Geometry check sheet. Reference: the model listing, model coordinates, mm. A direction names the side the tool comes from. Coordinates: 2 decimals unless noted, no trailing zeros. Loops run counter-clockwise (first coordinate to the right, second up) from the corner with the lowest first, then second, coordinate; pieces in that order, holes last.
Autodesk Fusion 360 part; units mm, degrees
sketch "Sketch1" plane through (0, 0, 0) normal (0, 0, 1) x (1, 0, 0)
  line L0 (0, 0) -> (-24.511, 0)
  line L1 (0, 0) -> (-1.1547, 2)
  line L2 (-1.1547, 2) -> (-3.1547, 2)
  line L3 (-3.1547, 2) -> (-4.6106, 6)
  line L4 (-4.6106, 6) -> (-4.9865, 5.8632)
  line L5 (-4.9865, 5.8632) -> (-3.5804, 2)
  line L6 (-3.5804, 2) -> (-4.1547, 2)
  line L7 (-4.5804, 2) -> (-5.1547, 2)
  line L8 (-5.9865, 5.8632) -> (-4.5804, 2)
  line L9 (-5.6106, 6) -> (-5.9865, 5.8632)
  line L10 (-4.1547, 2) -> (-5.6106, 6)
  line L11 (-5.5804, 2) -> (-6.1547, 2)
  line L12 (-6.9865, 5.8632) -> (-5.5804, 2)
  line L13 (-6.6106, 6) -> (-6.9865, 5.8632)
  line L14 (-5.1547, 2) -> (-6.6106, 6)
  line L15 (-6.5804, 2) -> (-7.1547, 2)
  line L16 (-7.9865, 5.8632) -> (-6.5804, 2)
  line L17 (-7.6106, 6) -> (-7.9865, 5.8632)
  line L18 (-6.1547, 2) -> (-7.6106, 6)
  line L19 (-7.5804, 2) -> (-8.1547, 2)
  line L20 (-8.9865, 5.8632) -> (-7.5804, 2)
  line L21 (-8.6106, 6) -> (-8.9865, 5.8632)
  line L22 (-7.1547, 2) -> (-8.6106, 6)
  line L23 (-8.5804, 2) -> (-9.1547, 2)
  line L24 (-9.9865, 5.8632) -> (-8.5804, 2)
  line L25 (-9.6106, 6) -> (-9.9865, 5.8632)
  line L26 (-8.1547, 2) -> (-9.6106, 6)
  line L27 (-9.1547, 2) -> (-12.9865, 2)
  line L28 (-20.9865, 10) -> (-20.9865, 0)
  line L29 (-12.9865, 2) -> (-12.9865, 10)
  line L30 (-12.9865, 10) -> (-20.9865, 10)
  line L31 (-12.9865, 2) -> (-12.9865, 0)
  line L32 (-9.6106, -6) -> (-9.9865, -5.8632)
  line L33 (-9.9865, -5.8632) -> (-8.5804, -2)
  line L34 (-7.1547, -2) -> (-8.6106, -6)
  line L35 (-5.1547, -2) -> (-6.6106, -6)
  line L36 (-9.1547, -2) -> (-12.9865, -2)
  line L37 (-7.5804, -2) -> (-8.1547, -2)
  line L38 (-3.5804, -2) -> (-4.1547, -2)
  line L39 (-20.9865, -10) -> (-20.9865, 0)
  line L40 (-12.9865, -10) -> (-20.9865, -10)
  line L41 (0, 0) -> (-1.1547, -2)
  line L42 (-4.9865, -5.8632) -> (-3.5804, -2)
  line L43 (-5.6106, -6) -> (-5.9865, -5.8632)
  line L44 (-6.5804, -2) -> (-7.1547, -2)
  line L45 (-7.6106, -6) -> (-7.9865, -5.8632)
  line L46 (-12.9865, -2) -> (-12.9865, -10)
  line L47 (-8.5804, -2) -> (-9.1547, -2)
  line L48 (-6.6106, -6) -> (-6.9865, -5.8632)
  line L49 (-12.9865, -2) -> (-12.9865, 0)
  line L50 (-7.9865, -5.8632) -> (-6.5804, -2)
  line L51 (-8.6106, -6) -> (-8.9865, -5.8632)
  line L52 (-6.1547, -2) -> (-7.6106, -6)
  line L53 (-4.6106, -6) -> (-4.9865, -5.8632)
  line L54 (-3.1547, -2) -> (-4.6106, -6)
  line L55 (-8.9865, -5.8632) -> (-7.5804, -2)
  line L56 (-8.1547, -2) -> (-9.6106, -6)
  line L57 (-6.9865, -5.8632) -> (-5.5804, -2)
  line L58 (-4.1547, -2) -> (-5.6106, -6)
  line L59 (-1.1547, -2) -> (-3.1547, -2)
  line L60 (-5.9865, -5.8632) -> (-4.5804, -2)
  line L61 (-4.5804, -2) -> (-5.1547, -2)
  line L62 (-5.5804, -2) -> (-6.1547, -2)
  line L63 (-14.4865, 2) -> (-14.4865, 0)
  line L64 (-14.4865, -2) -> (-14.4865, 0)
  line L65 (-14.4865, -2) -> (-14.4865, -8.5)
  line L66 (-14.4865, -8.5) -> (-19.4865, -8.5)
  line L67 (-19.4865, -8.5) -> (-19.4865, 0)
  line L68 (-19.4865, 8.5) -> (-19.4865, 0)
  line L69 (-14.4865, 8.5) -> (-19.4865, 8.5)
  line L70 (-14.4865, 2) -> (-14.4865, 8.5)
  point P0 (-24.511, 0)
  dimension "d1" = 4
  dimension "d2" = 0.4
  dimension "d3" = 1
  dimension "d6" = -1
  dimension "d7" = 0
  dimension "d8" = 110
  dimension "d9" = 4
  dimension "d10" = 8
  dimension "d11" = 8
  dimension "d12" = 3
  dimension "d13" = 2
  dimension "d14" = 60
  dimension "d19" = 1.5
extrude "Extrude1" add sketch "Sketch1" along normal blind 3 contours L0 L1 L2 L3 L4 L5 L6 L7 L8 L9 L10 L11 L12 L13 L14 L15 L16 L17 L18 L19 L20 L21 L22 L23 L24 L25 L26 L27 L31
extrude "Extrude2" add sketch "Sketch1" along normal blind 10 contours L0 L39 L40 L46 L49 L64 L65 L66 L67 | L0 L28 L29 L30 L31 L63 L68 L69 L70
(1) Sectioned sample at A-A on y = -7.5. Record the cut outline in (x, z), and give its area (3 significant figures).
Findings:
outline: (-20.99, 0) - (-19.49, 0) - (-19.49, 10) - (-20.99, 10) - close; (-14.49, 0) - (-12.99, 0) - (-12.99, 10) - (-14.49, 10) - close
area: 30.0 mm2
(2) Scan lines: L1, parallel to X at y = 2, z = 4; L2, parallel to Y at x = -15.75, z = 3.5; L3, parallel to Y at x = -2.75, z = 2.75. Record each from-to range of solid material in increasing order.
Findings:
L1: x = -20.99 to -19.49, -14.49 to -12.99
L2: y = -10 to -8.5, 8.5 to 10
L3: y = 0 to 2
(3) Sectioned sample at B-B on z = 5.75. Record the cut outline in (x, y).
Findings:
outline: (-20.99, -10) - (-12.99, -10) - (-12.99, 10) - (-20.99, 10) - close; hole (-19.49, -8.5) - (-14.49, -8.5) - (-14.49, 8.5) - (-19.49, 8.5) - close
(4) Sectioned sample at C-C on x = -18.75. Record the cut outline in (y, z), and give its area (3 significant figures).
Findings:
outline: (-10, 0) - (-8.5, 0) - (-8.5, 10) - (-10, 10) - close; (8.5, 0) - (10, 0) - (10, 10) - (8.5, 10) - close
area: 30.0 mm2
(5) Access from +Z, -Z, +X, -X, +Y, -Y to the whole of each face (thin tool, end or side, straight path). Record for faces 1 (the flat face through (-8.87, 3.97, 1.48)), 2 (the flat face through (-2, 2, 1)), 3 (the flat face through (-17, 10, 5)).
Findings:
face 1: +Z, -Z
face 2: +Z, -Z, +X, +Y
face 3: +Z, -Z, +X, -X, +Y
(6) Draft check along Y on faces 4 (the flat face through (-4.293, 3.959, 1.479)), 5 (the flat face through (-17, -10, 5)), 6 (the flat face through (-9.293, 3.959, 1.479)), 7 (the flat face through (-14, 0, 10)). Enter one of: +Y half, -Y half, draft (parallel to the pull), parting line (faces both ways), or undercut.
Findings:
face 4: undercut
face 5: -Y half
face 6: undercut
face 7: draft
(7) Gauge pin test, flat ends, axial feed: pin 1 Ø3 at (x, y) = (-8.5, 2.5) entering from +Z; pin 2 Ø2.5 at (x, z) = (-11, 1) entering from +Y; pin 3 Ø3 at (y, z) = (4, 4) entering from +X. Record the tip position at first contact, or that the pin passes through.
Findings:
pin 1: stops at z = 3
pin 2: stops at y = 5.95
pin 3: stops at x = -3.48
(8) Sectioned sample at D-D on y = 1.5. Record the cut outline in (x, z).
Findings:
outline: (-20.99, 0) - (-19.49, 0) - (-19.49, 10) - (-20.99, 10) - close; (-14.49, 0) - (-0.87, 0) - (-0.87, 3) - (-12.99, 3) - (-12.99, 10) - (-14.49, 10) - close
